The drawing under review shows one solid part. Ordinate dimensions are in mm from its lowest x, y, z. A direction names the side the tool comes from. Round coordinates to 2 decimals unless told otherwise and drop trailing zeros. Write each loop counter-clockwise with the first axis right and the second up, starting at its lowest first coordinate (ties: lowest second). Pieces come first, ordered by that corner, then holes.
Item 1: Clearance check with flat-ended pins moving along their axes: pin 1 Ø0.6 at (x, z) = (8.5, 2.5) entering from +Y; pin 2 Ø2 at (y, z) = (5.5, 1.5) entering from -X; pin 3 Ø6 at (x, y) = (5, 6) entering from -Z. State where each tip first meets the part, or that it passes through.
Item 2: To check wall thickness, follow L1, parallel to Y at x = 5, z = 14.6; L2, parallel to Z at x = 2, y = 7; L3, parallel to Z at x = 5.5, y = 3. State the ranges of each line that lie inside material, in increasing order.
Item 3: Add section C-C (y = 4.25). Give the boundary of the cut face in (x, z).
Item 4: Machinability: for the marked faces 1, 2, 3, 4 and 5, which of the approach directions +Z, -Z, +X, -X, +Y, -Y give a long, thin tool a straight path to every point of the face, cutting with its end or side? Answer none if there is none.
Item 5: Add section B-B (x = 5). Give the boundary of the cut face in (y, z).
Item 6: Add section D-D (z = 8). Give the boundary of the cut face in (x, y).
Item 7: Draft analysis for pull direction X (two halves, no side actions). For the marked faces 6, 7 and 8, state which applies: +X half, -X half, draft (parallel to the pull), parting line (faces both ways), or undercut.
Item 8: Add section A-A (z = 13.75). Give the boundary of the cut face in (x, y), plus the area to 3 significant figures.
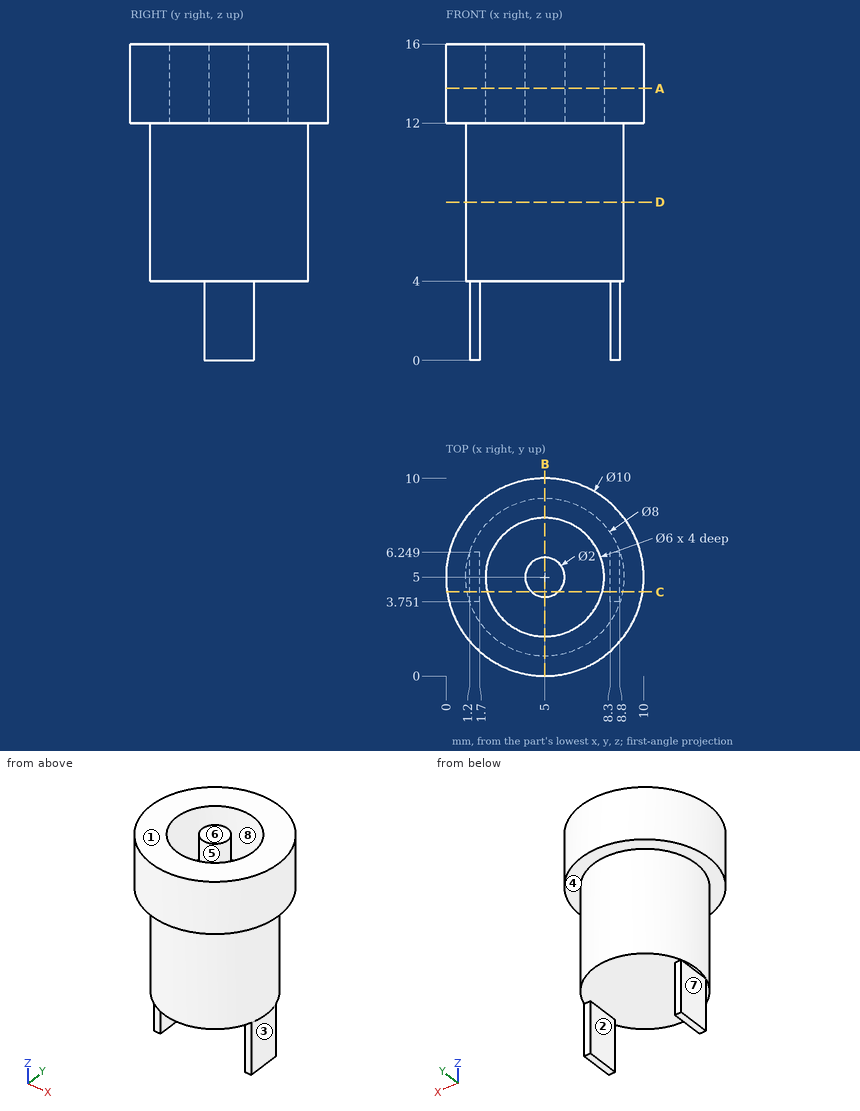
Numbers:
1. pin 1: stops at y = 6.25
1. pin 2: stops at x = 1.2
1. pin 3: stops at z = 4
2. L1: y = 0 to 2, 4 to 6, 8 to 10
2. L2: z = 4 to 16
2. L3: z = 4 to 12
3. outline: (0.06, 12) - (1.07, 12) - (1.07, 4) - (1.2, 4) - (1.2, 0) - (1.7, 0) - (1.7, 4) - (8.3, 4) - (8.3, 0) - (8.8, 0) - (8.8, 4) - (8.93, 4) - (8.93, 12) - (9.94, 12) - (9.94, 16) - (7.9, 16) - (7.9, 12) - (5.66, 12) - (5.66, 16) - (4.34, 16) - (4.34, 12) - (2.1, 12) - (2.1, 16) - (0.06, 16) - close
4. face 1: +Z, +X, -X, +Y, -Y
4. face 2: -Z, +Y, -Y
4. face 3: -Z, +X, +Y, -Y
4. face 4: -Z
4. face 5: +Z
5. outline: (0, 12) - (1, 12) - (1, 4) - (9, 4) - (9, 12) - (10, 12) - (10, 16) - (8, 16) - (8, 12) - (6, 12) - (6, 16) - (4, 16) - (4, 12) - (2, 12) - (2, 16) - (0, 16) - close
6. outline: circle Ø8 at (5, 5)
7. face 6: draft
7. face 7: -X half
7. face 8: undercut
8. outline: circle Ø10 at (5, 5); circle Ø2 at (5, 5); hole circle Ø6 at (5, 5)
8. area: 53.4 mm2
